Could you check a few things on this model? Use its own coordinates, in mm. Give positions to 0.01 mm unless a question says otherwise; leave off trailing zeros. Write each loop counter-clockwise with the first axis right and the second up, starting at its lowest first coordinate (ties: lowest second). Pieces come first, ordered by that corner, then holes. Notation, with made-up numbers: (-27, 1.25) -> (10, 1.25) arc R8 cw to (10, 9.25) -> close; hole circle Ø11 at (15.25, 59.5). An arc over 180 degrees is marked (long way). Write item = value, one per line. Start each with the question number.
```python
from build123d import *

# Parameters (mm, degrees)
SKETCH3_R           = 0.889
BOSS_EXTRUDE1_DEPTH = 9.525
CHAMFER1_SIZE       = 0.254
CUT_EXTRUDE1_START  = 0.254
SKETCH4_W           = 0.8128
SKETCH4_H           = 4.2418
CUT_EXTRUDE1_DEPTH  = 10.732093261


with BuildPart() as part:
    # Sketch2 → Revolve1 (revolve)
    with BuildSketch(Plane(origin=(0, 0, 0), x_dir=(0, 0, -1), z_dir=(1, 0, 0))):
        with BuildLine():
            Line((0, 0), (2.1209, 0))
            ThreePointArc((2.1209, 0), (1.320815264, 1.138053219), (0, 1.5748))
            Line((0, 1.5748), (0, 0))
        make_face()
    revolve(axis=Axis((0, 0.415157056, 0), (0, -1, 0)))

    # Sketch3 → Boss-Extrude1 (add)
    with BuildSketch(Plane.XZ):
        with Locations(Location((0, 0, 0), (0, 0, 90))):
            Circle(SKETCH3_R)
    extrude(amount=BOSS_EXTRUDE1_DEPTH)

    # Chamfer1
    chamfer1_edges = [part.edges().sort_by_distance(p)[0] for p in [
        (0, -9.525, -0.889),
    ]]
    chamfer(chamfer1_edges, length=CHAMFER1_SIZE)

    # Sketch4 → Cut-Extrude1 (cut, through all)
    with BuildSketch(Plane(origin=(0, 0, 0), x_dir=(1, 0, 0), z_dir=(0, 1, 0)).offset(CUT_EXTRUDE1_START)):
        Rectangle(SKETCH4_W, SKETCH4_H)
    extrude(amount=CUT_EXTRUDE1_DEPTH, mode=Mode.SUBTRACT)


solid = part.part
```
(1) I'm going to push flat-ended pins straight in: pin 1 (1.5 mm diameter, centred on x = -1, y = -6.5, fed in from +Z); pin 2 (1.4 mm diameter, centred on y = 0.5, z = 1, fed in from -X); pin 3 (0.6 mm diameter, centred on y = 1, z = 0, fed in from +X). Where does each tip first touch, or does it pass through?
(2) We'd pull the mould along X, two halves only. Please class faces 1 (the flat face through (0, -9.525, 0)), 2 (the flat face through (-0.406, 1, 0)), 3 (the cylindrical face through (0.87, -4.57, -0.19)): released by +X, released by -X, zero draft, split by the parting line, or undercut.
(3) Imagine slicing it at C-C (y = -6.5). Please give me the cut outline in (x, z), then the cut area to 3 significant figures.
(4) If I drill on line 1 along X through (y, z) = (-8.5, 0.05); line 2 along Y through (x, z) = (0.25, 0.1) (3 decimals); line 3 along Y through (x, z) = (0.25, 1.7), over which ranges is the centre line in solid material (lowest first)? Write a range as from..to.
(5) Imagine slicing it at B-B (z = 0). Please give me the cut outline in (x, y) (3 decimals), then the cut area to 3 significant figures.
(6) Imagine slicing it at A-A (x = 0). Please give me the cut outline in (y, z) (3 decimals).
Answers below:
q1.pin_1 = 0.85
q1.pin_2 = -2.06
q1.pin_3 = 1.76
q2.face_1 = zero draft
q2.face_2 = undercut
q2.face_3 = split by the parting line
q3.outline = circle Ø1.78 at (0, 0)
q3.area = 2.48 mm^2
q4.line_1 = -0.89..0.89
q4.line_2 = -9.525..0.254
q4.line_3 = 0..0.25
q5.outline = (-2.121, 0) -> (-0.889, 0) -> (-0.889, -9.271) -> (-0.635, -9.525) -> (0.635, -9.525) -> (0.889, -9.271) -> (0.889, 0) -> (2.121, 0) arc R2.216 ccw to (0.406, 1.537) -> (0.406, 0.254) -> (-0.406, 0.254) -> (-0.406, 1.537) arc R2.216 ccw to start
q5.area = 20.7 mm^2
q6.outline = (-9.525, -0.635) -> (-9.271, -0.889) -> (0, -0.889) -> (0, -2.121) arc R2.216 ccw to (0.254, -2.027) -> (0.254, 2.027) arc R2.216 ccw to (0, 2.121) -> (0, 0.889) -> (-9.271, 0.889) -> (-9.525, 0.635) -> close
